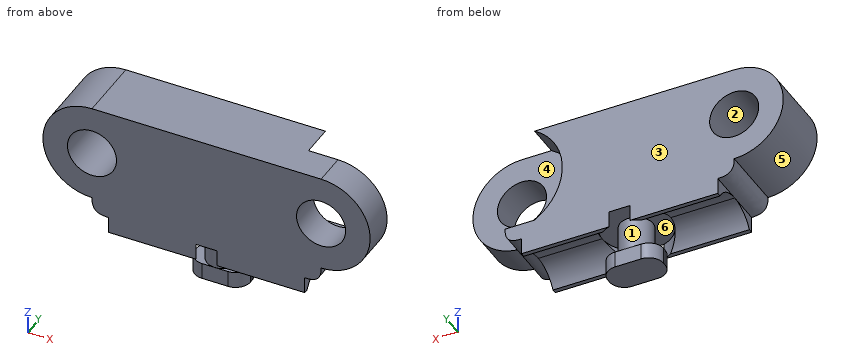
from build123d import *

# Parameters (mm, degrees)
SKETCH1_R                = 1.5
BOSS_EXTRUDE1_DEPTH      = 2
CUT_EXTRUDE1_DEPTH       = 2
BOSS_EXTRUDE2_REACH      = 13.18
SKETCH3_W                = 14
SKETCH3_H                = 1
FILLET1_SIZE             = 1
BOSS_EXTRUDE3_DEPTH      = 6
BOSS_EXTRUDE3_DEPTH_BACK = 6
CUT_EXTRUDE4_START       = -4
SKETCH5_R                = 2.1
CUT_EXTRUDE4_DEPTH       = 10
SKETCH6_R                = 1
BOSS_EXTRUDE5_DEPTH      = 3
BOSS_EXTRUDE6_START      = 2
BOSS_EXTRUDE6_DEPTH      = 1


with BuildPart() as part:
    # Sketch1 → Boss-Extrude1 (new, symmetric)
    with BuildSketch(Plane(origin=(0, 0, 0), x_dir=(1, 0, 0), z_dir=(0, 1, 0))):
        with BuildLine():
            Line((-7, 3), (7, 3))
            ThreePointArc((7, 3), (10, 0), (7, -3))
            Line((7, -3), (-7, -3))
            ThreePointArc((-7, -3), (-10, 0), (-7, 3))
        make_face()
        with Locations(Location((-7, 0, 0), (0, 0, 270))):
            Circle(SKETCH1_R, mode=Mode.SUBTRACT)
        with Locations(Location((7, 0, 0), (0, 0, 270))):
            Circle(SKETCH1_R, mode=Mode.SUBTRACT)
    extrude(amount=BOSS_EXTRUDE1_DEPTH, both=True)

    # Sketch2 → Cut-Extrude1 (cut)
    with BuildSketch(Plane(origin=(0, 2, 0), x_dir=(1, 0, 0), z_dir=(0, 1, 0))):
        with BuildLine():
            Line((5.197224362, 3), (7, 3))
            ThreePointArc((7, 3), (10, 0), (7, -3))
            Line((7, -3), (5.197224362, -3))
            ThreePointArc((5.197224362, -3), (3.5, 0), (5.197224362, 3))
        make_face()
    extrude(amount=-CUT_EXTRUDE1_DEPTH, mode=Mode.SUBTRACT)

    # Boss-Extrude2: up to this face of the body (flat: up to its plane)
    boss_extrude2_end = Plane(part.part.faces().sort_by_distance((-2.270949872, 2, 0))[0])
    # Sketch3 → Boss-Extrude2 (add, up to the picked face)
    with BuildSketch(Plane.XZ.offset(2), mode=Mode.PRIVATE) as boss_extrude2_sk1:
        with Locations((0, -3.5)):
            Rectangle(SKETCH3_W, SKETCH3_H)
    boss_extrude2_tool1 = split(extrude(boss_extrude2_sk1.sketch, amount=-BOSS_EXTRUDE2_REACH, mode=Mode.PRIVATE), bisect_by=boss_extrude2_end, keep=Keep.BOTH, mode=Mode.PRIVATE)
    add(boss_extrude2_tool1.solids().sort_by(Axis((0, -2, -3.5), (0, 1, 0)))[0])

    # Fillet1
    # a fillet whose section is not a circle: 1 mm, written as the material it takes off along each edge
    with BuildSketch(Plane(origin=(7, -4.5, -4), x_dir=(0, 0, 1), z_dir=(0, 1, 0)), Plane(origin=(-7, -4.5, -4), x_dir=(1, 0, 0), z_dir=(0, 1, 0))) as fillet1_piece_1:
        with BuildLine():
            add(Edge.make_bspline([(FILLET1_SIZE, 0), (FILLET1_SIZE * 0.831801948466, 0), (FILLET1_SIZE * 0.663603896932, 0), (FILLET1_SIZE * 0.292893218813, -FILLET1_SIZE * 0.0716919198361), (FILLET1_SIZE * 0.0716919198361, -FILLET1_SIZE * 0.292893218813), (0, -FILLET1_SIZE * 0.663603896932), (0, -FILLET1_SIZE * 0.831801948466), (0, -FILLET1_SIZE)], knots=[0, 0, 0, 0, 0, 0, 0.5, 0.5, 1, 1, 1, 1, 1, 1], degree=5))
            Line((0, -FILLET1_SIZE), (0, 0))
            Line((0, 0), (FILLET1_SIZE, 0))
        make_face()
    extrude(amount=9, mode=Mode.SUBTRACT)

    # Sketch4 → Boss-Extrude3 (add, two sides: drawn at the far end of the back side and taken through both)
    with BuildSketch(Plane(origin=(0, 0, 0), x_dir=(0, 0, -1), z_dir=(1, 0, 0)).offset(-BOSS_EXTRUDE3_DEPTH_BACK)):
        with BuildLine():
            Line((5, 2), (4, 2))
            Line((4, 2), (4, 0))
            ThreePointArc((4, 0), (4.267949192, 1), (5, 1.732050808))
            Line((5, 1.732050808), (5, 2))
        make_face()
        with BuildLine():
            ThreePointArc((5, -1.732050808), (4.267949192, -1), (4, 0))
            Line((4, 0), (4, -2))
            Line((4, -2), (5, -2))
            Line((5, -2), (5, -1.732050808))
        make_face()
    extrude(amount=BOSS_EXTRUDE3_DEPTH + BOSS_EXTRUDE3_DEPTH_BACK)

    # Sketch5 → Cut-Extrude4 (cut)
    with BuildSketch(Plane.XY.offset(CUT_EXTRUDE4_START)):
        Circle(SKETCH5_R)
    extrude(amount=-CUT_EXTRUDE4_DEPTH, mode=Mode.SUBTRACT)

    # Sketch6 → Boss-Extrude5 (add)
    with BuildSketch(Plane(origin=(0, 0, -4), x_dir=(-1, 0, 0), z_dir=(0, 0, -1))):
        with Locations(Location((0, 0, 0), (0, 0, 180))):
            Circle(SKETCH6_R)
    extrude(amount=BOSS_EXTRUDE5_DEPTH)

    # Sketch6<3> → Boss-Extrude6 (add)
    with BuildSketch(Plane(origin=(0, 0, -4), x_dir=(-1, 0, 0), z_dir=(0, 0, -1)).offset(BOSS_EXTRUDE6_START)):
        with BuildLine():
            Line((0.8, 1), (0, 1))
            ThreePointArc((0, 1), (0.707106781, 0.707106781), (1, 0))
            ThreePointArc((1, 0), (0.707106781, -0.707106781), (0, -1))
            Line((0, -1), (0.8, -1))
            ThreePointArc((0.8, -1), (1.436396103, -0.736396103), (1.7, -0.1))
            Line((1.7, -0.1), (1.7, 0.1))
            ThreePointArc((1.7, 0.1), (1.436396103, 0.736396103), (0.8, 1))
        make_face()
        with BuildLine():
            ThreePointArc((0, -1), (-1, 0), (0, 1))
            Line((0, 1), (-0.8, 1))
            ThreePointArc((-0.8, 1), (-1.436396103, 0.736396103), (-1.7, 0.1))
            Line((-1.7, 0.1), (-1.7, -0.1))
            ThreePointArc((-1.7, -0.1), (-1.436396103, -0.736396103), (-0.8, -1))
            Line((-0.8, -1), (0, -1))
        make_face()
    extrude(amount=BOSS_EXTRUDE6_DEPTH)


solid = part.part
Can you work these out from the model? Positions are in its coordinate system, mm. Face numbers are marked on the shaded views. A direction names the side the tool comes from. Coordinates: 2 decimals unless noted, no trailing zeros. Write each loop counter-clockwise with the first axis right and the second up, starting at its lowest first coordinate (ties: lowest second). Pieces come first, ordered by that corner, then holes. Notation, with made-up numbers: (-30.75, 35) -> (4.25, 35) arc R12 ccw to (4.25, 43) -> close; hole circle Ø8 at (79, 48). An arc over 180 degrees is marked (long way). Write each question's results on one line, items separated by ' | '. Start each with the question number.
Item 1: Please list where these lines run through material, in increasing order: probe 1 along X at (y, z) = (-1.2, 0); probe 2 along X at (y, z) = (0.9, 0); probe 3 along X at (y, z) = (-1.5, -0.5).
Item 2: On a 3-axis mill with a long thin cutter (end or side, diameter ignored), from which of +Z, -Z, +X, -X, +Y, -Y can I reach the whole of each face in a straight line? I mean the marked faces 4, 5 and 6. Say none if no direction works.
Item 3: Thinking about a two-plate mould opening in Y: for the marked faces 1, 2 and 3, which applies, released by +Y, released by -Y, zero draft, split by the parting line, or undercut?
Item 4: I'm going to push flat-ended pins straight in: P1, Ø0.5, axis at x = 6, y = 0.5, coming from the +Z side; P2, Ø1.5, axis at x = -7.5, y = -1, coming from the +Z side; P3, Ø5, axis at x = 7.5, z = -0.5, coming from the +Y side; P4, Ø0.5, axis at y = -1, z = -4.5, coming from the -X side. Where does each tip first touch, or does it pass through?
Item 5: If we section it at A-A, the plane z = 0: Write out the boundary of the cut face in (x, y), and give its area (3 significant figures).
Item 6: If we section it at B-B, the plane x = -5.75: Write out the boundary of the cut face in (y, z).
Item 7: If we section it at D-D, the plane z = 2: Write out the boundary of the cut face in (x, y), and give its area (3 significant figures).
Item 8: If we section it at C-C, the plane x = 3.25: Write out the boundary of the cut face in (y, z).
Answer block:
1) probe 1: -10 to -8.5, -5.5 to 5.5, 8.5 to 10 | probe 2: -10 to -8.5, -5.5 to 3.5 | probe 3: -9.96 to -8.41, -5.59 to 5.59, 8.41 to 9.96
2) face 4: +X, +Y | face 5: -X, +Y, -Y | face 6: none
3) face 1: undercut | face 2: zero draft | face 3: released by +Y
4) P1: z = -3 | P2: z = 3 | P3: y = 0 | P4: x = -6
5) outline: (-10, -2) -> (-8.5, -2) -> (-8.5, 2) -> (-10, 2) -> close; (-5.5, -2) -> (5.5, -2) -> (5.5, 0) -> (3.5, 0) -> (3.5, 2) -> (-5.5, 2) -> close; (8.5, -2) -> (10, -2) -> (10, 0) -> (8.5, 0) -> close | area: 49.0 mm²
6) outline: (-2, -5) -> (-1.73, -5) arc R2 cw to (1.73, -5) -> (2, -5) -> (2, -0.83) -> (-2, -0.83) -> close; (-2, 0.83) -> (2, 0.83) -> (2, 3) -> (-2, 3) -> close
7) outline: (-9.24, -2) -> (9.24, -2) -> (9.24, 0) -> (4.13, 0) -> (4.13, 2) -> (-9.24, 2) -> close | area: 63.7 mm²
8) outline: (-2, -5) -> (-1.73, -5) arc R2 cw to (1.73, -5) -> (2, -5) -> (2, 3) -> (-2, 3) -> close
